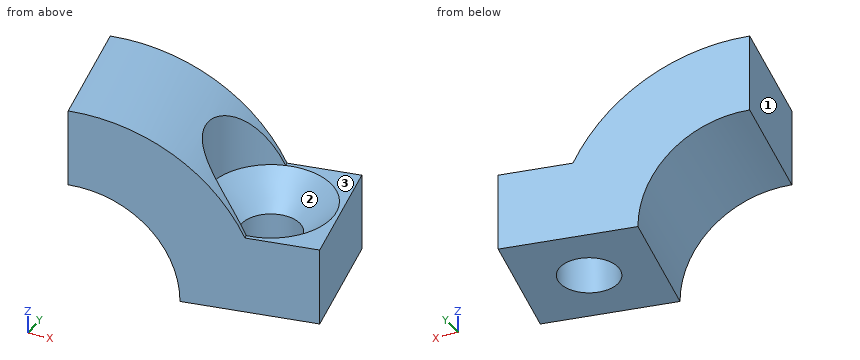
```python
from build123d import *

# Parameters (mm, degrees)
EXTRUDE_1_DEPTH     = 5
CUT_EXTRUDE_1_REACH = 109.797
SKETCH_2_R          = 4.7


# Read off the part's stored shape, not the designer's step: 高级异型孔1
with BuildPart() as part:
    # 草图1 → 凸台-拉伸1 (new, symmetric)
    with BuildSketch(Plane(origin=(-126.798228997, -64.222453956, -29.938468974), x_dir=(0, 0, -1), z_dir=(-0.21174441426742976, 0.9773250754107066, 0))):
        with BuildLine():
            Line((-40, -48), (-40, -58))
            Line((-40, -58), (-46, -58))
            Line((-46, -58), (-46, -52.649110641))
            ThreePointArc((-46, -52.649110641), (-51.832159566, -47.483314774), (-54, -40))
            Line((-54, -40), (-48, -40))
            ThreePointArc((-48, -40), (-45.656854249, -45.656854249), (-40, -48))
        make_face()
    extrude(amount=EXTRUDE_1_DEPTH, both=True)

    # 高级异型孔1 outline → 高级异型孔1 (revolve, cut)
    with BuildSketch(Plane(origin=(-75, -53, 0), x_dir=(1, 0, 0), z_dir=(0, -1, 0))):
        Polygon((0, 10.061531026), (2.25, 10.061531026), (2.25, 13.611531026), (4.7, 16.061531026), (0, 16.061531026), align=None)
    revolve(axis=Axis((-75, -53, 0), (0, 0, 1)), mode=Mode.SUBTRACT)

    # 草图2 → 切除-拉伸1 (cut, up to next)
    with BuildSketch(Plane.XY.offset(16.061531026), mode=Mode.PRIVATE) as cut_extrude_1_sk1:
        with Locations((-75, -53)):
            Circle(SKETCH_2_R)
    cut_extrude_1_tool1 = extrude(cut_extrude_1_sk1.sketch, amount=CUT_EXTRUDE_1_REACH, mode=Mode.PRIVATE) & part.part
    add(cut_extrude_1_tool1.solids().sort_by_distance((-75, -53, 16.061531))[0], mode=Mode.SUBTRACT)


solid = part.part
```
Work out the finished part from the listing and answer in its coordinate system (mm). Face numbers are marked on the shaded views. Give positions to 0.01 mm unless a question says otherwise; leave off trailing zeros. Loops run counter-clockwise (first coordinate to the right, second up) from the corner with the lowest first, then second, coordinate; pieces in that order, holes last. Notation, with made-up numbers: (79.25, -21.5) -> (99.25, -21.5) arc R32 ccw to (99.25, 16.5) -> close; hole circle Ø10 at (4, 26.5). An arc over 180 degrees is marked (long way). Put each result on its own line as item: value. Start each with the question number.
Item 1: The part is cut by section A-A (z = 14). Give the vertices of the cut face in (x, y), then the cut area to 3 significant figures.
Item 2: The part is cut by section C-C (z = 12.5). Give the vertices of the cut face in (x, y).
Item 3: Find the intervals of material crossed by L1, parallel to Z at x = -71, y = -49.25; L2, parallel to Y at x = -75, z = 11.7; L3, parallel to X at y = -51.25, z = 14.25, in increasing order. Write a range as [from, to].
Item 4: The part is cut by section B-B (z = 20). Give the vertices of the cut face in (x, y), then the cut area to 3 significant figures.
Item 5: The part is cut by section D-D (z = 17). Give the vertices of the cut face in (x, y).
Item 6: Each of these flat-tipped pins is pushed along its axis until it touches: P1, Ø3, axis at y = -55.5, z = 21.5, coming from the +X side; P2, Ø3.5, axis at x = -73, y = -51, coming from the +Z side; P3, Ø1, axis at x = -79.5, z = 17, coming from the -Y side. Where does it stop, or does it pass through?
Item 7: The mould has two halves that part along Y. Classify the marked faces 1, 2 and 3: released by +Y, released by -Y, zero draft, split by the parting line, or undercut.
Answers below:
1. outline: (-81.96, -49.39) -> (-79.84, -59.16) -> (-69.05, -56.83) -> (-71.17, -47.05) -> close; hole circle Ø5.28 at (-75, -53)
1. area: 88.5 mm2
2. outline: (-81.32, -49.25) -> (-79.2, -59.03) -> (-69.05, -56.83) -> (-71.17, -47.05) -> close; hole circle Ø4.5 at (-75, -53)
3. L1: [10.06, 16.06]
3. L2: [-58.12, -55.25], [-50.75, -47.88]
3. L3: [-81.71, -77.3], [-72.7, -70.26]
4. outline: (-88.76, -50.87) -> (-86.65, -60.64) -> (-77.01, -58.55) -> (-77.33, -57.08) arc R4.7 cw to (-78.81, -50.25) -> (-79.13, -48.78) -> close
4. area: 91.0 mm2
5. outline: (-84.87, -50.02) -> (-82.75, -59.8) -> (-74.76, -58.06) -> (-74.84, -57.7) arc R4.7 cw to (-76.8, -48.66) -> (-76.88, -48.29) -> close
6. P1: x = -77.99
6. P2: z = 15.94
6. P3: y = -59.2
7. face 1: released by -Y
7. face 2: undercut
7. face 3: zero draft
